For this review, take the finished solid that the model builds, in its own axes (mm). A direction names the side the tool comes from. Coordinates: 2 decimals unless noted, no trailing zeros. Loops run counter-clockwise (first coordinate to the right, second up) from the corner with the lowest first, then second, coordinate; pieces in that order, holes last. Notation, with made-up numbers: M 24.5,-27 L 57.5,-27 A18 cw 57.5,8 Z; hole C -25,-36.5 d10. An arc over 180 degrees is marked long. Answer as a JSON object with one key per item and string values. Group by question number.
Item 1: Add section A-A (z = 35.5). State the section outline as (x, y) points, then the cut area to 3 significant figures.
Item 2: Add section B-B (y = 3). State the section outline as (x, z) points.
Item 3: Mouldability with a two-part tool opening along Z and no side actions: class faces 1 (the face through (-47.435, -1, 35)), 2 (the face through (-1, 1, 11.176)), 3 (the face through (0.593, -61.131, 1.528)) as +Z half, -Z half, draft (parallel to the pull), parting line (faces both ways), or undercut.
Item 4: Wall thickness on L1, parallel to Y at x = -34.5, z = 60; L2, parallel to X at y = 52.5, z = 63.5; L3, parallel to Z at x = -3, y = -27.5: over which ranges is each line inside the solid? List them lowest first. Write a range as from..to.
Item 5: Tool access review of faces 4 (the face through (37.719, -1, 41)), 5 (the face through (-1, 62.579, 35)): name each direction out of +Z, -Z, +X, -X, +Y, -Y from which nothing blocks a thin tool from reaching the whole face with its end or side.
Item 6: Insertion check: pin 1 (1.5 mm diameter, centred on x = 34, y = -3, fed in from +Z). The pin has a flat end and moves straight along its axis. Give the tip position at first contact, or say it passes through.
Item 7: Add section C-C (x = -23). State the section outline as (y, z) points.
from build123d import *

# Parameters (mm, degrees)
F0_W     = 94.869002
F0_H     = 125.158504
F1_DEPTH = 70.358
F2_W     = 75.438
F2_H     = 106.870502
F3_DEPTH = 59.182
F4_R     = 5.08


with BuildPart() as f1:
    # F0 (on Top) → F1 (new body)
    with BuildSketch(Plane.XY):
        Rectangle(F0_W, F0_H)
    extrude(amount=F1_DEPTH)

    # F2 (on face) → F3 (cut)
    with BuildSketch(Plane.XY.offset(70.358)):
        Rectangle(F2_W, F2_H)
    extrude(amount=-F3_DEPTH, mode=Mode.SUBTRACT)

    # F4
    f4_edges = [f1.edges().sort_by_distance(p)[0] for p in [
        (47.434501, 62.579252, 35.179),
        (0, 62.579252, 70.358),
        (-47.434501, 0, 70.358),
        (0, -62.579252, 70.358),
        (47.434501, -62.579252, 35.179),
        (47.434501, 0, 0),
        (47.434501, 0, 70.358),
        (-47.434501, -62.579252, 35.179),
        (0, -62.579252, 0),
        (-47.434501, 62.579252, 35.179),
        (-47.434501, 0, 0),
        (0, 62.579252, 0),
    ]]
    fillet(f4_edges, radius=F4_R)


solid = f1.part
From the geometry:
{
 "1": {"outline": "M -47.43,-57.5 A5.08 ccw -42.35,-62.58 L 42.35,-62.58 A5.08 ccw 47.43,-57.5 L 47.43,57.5 A5.08 ccw 42.35,62.58 L -42.35,62.58 A5.08 ccw -47.43,57.5 Z; hole M -37.72,-53.44 L 37.72,-53.44 L 37.72,53.44 L -37.72,53.44 Z", "area": "3,790 mm²"},
 "2": {"outline": "M -47.43,5.08 A5.08 ccw -42.35,0 L 42.35,0 A5.08 ccw 47.43,5.08 L 47.43,65.28 A5.08 ccw 42.35,70.36 L 37.72,70.36 L 37.72,11.18 L -37.72,11.18 L -37.72,70.36 L -42.35,70.36 A5.08 ccw -47.43,65.28 Z"},
 "3": {"face 1": "draft", "face 2": "+Z half", "face 3": "-Z half"},
 "4": {"L1": "y = -62.58..-53.44, 53.44..62.58", "L2": "x = -47.43..-37.72, 37.72..47.43", "L3": "z = 0..11.18"},
 "5": {"face 4": "+Z", "face 5": "+Z, -Z, +X, -X, +Y"},
 "6": {"pin 1": "stops at z = 11.18"},
 "7": {"outline": "M -62.58,5.08 A5.08 ccw -57.5,0 L 57.5,0 A5.08 ccw 62.58,5.08 L 62.58,65.28 A5.08 ccw 57.5,70.36 L 53.44,70.36 L 53.44,11.18 L -53.44,11.18 L -53.44,70.36 L -57.5,70.36 A5.08 ccw -62.58,65.28 Z"}
}
